```python
from build123d import *

# Parameters (mm, degrees)
SKETCH_1_W          = 15
SKETCH_1_H          = 15
SKETCH_1_W_2        = 12
SKETCH_1_H_2        = 12
EXTRUDE_1_DEPTH     = 267.5
SKETCH_2_R          = 2.15
CUT_EXTRUDE_1_DEPTH = 269.025185384
SKETCH_3_R          = 2.15
CUT_EXTRUDE_2_DEPTH = 269.025185384


with BuildPart() as part:
    # ｽｹｯﾁ1 → 押し出し-薄板1 (new body)
    with BuildSketch(Plane(origin=(0, 0, 0), x_dir=(1, 0, 0), z_dir=(0, 1, 0))):
        Rectangle(SKETCH_1_W, SKETCH_1_H)
        Rectangle(SKETCH_1_W_2, SKETCH_1_H_2, mode=Mode.SUBTRACT)
    extrude(amount=EXTRUDE_1_DEPTH)

    # ｽｹｯﾁ2 → ｶｯﾄ - 押し出し1 (cut, through all)
    with BuildSketch(Plane.ZY.offset(-7.5)):
        with Locations(Location((0, 5, 0), (0, 0, 180))):
            Circle(SKETCH_2_R)
        with Locations(Location((0, 262.5, 0), (0, 0, 180))):
            Circle(SKETCH_2_R)
        with Locations(Location((0, 250, 0), (0, 0, 180))):
            Circle(SKETCH_2_R)
    extrude(amount=CUT_EXTRUDE_1_DEPTH, mode=Mode.SUBTRACT)

    # ｽｹｯﾁ3 → ｶｯﾄ - 押し出し2 (cut, through all)
    with BuildSketch(Plane.XY.offset(7.5)):
        with Locations((0, 207.5)):
            Circle(SKETCH_3_R)
        with Locations((0, 232.5)):
            Circle(SKETCH_3_R)
        with Locations((0, 65)):
            Circle(SKETCH_3_R)
        with Locations((0, 40)):
            Circle(SKETCH_3_R)
    extrude(amount=-CUT_EXTRUDE_2_DEPTH, mode=Mode.SUBTRACT)


solid = part.part
```
The model under review builds one solid part; all positions refer to its coordinate system, in mm. A direction names the side the tool comes from. Give positions to 0.01 mm unless a question says otherwise; leave off trailing zeros. Write each loop counter-clockwise with the first axis right and the second up, starting at its lowest first coordinate (ties: lowest second). Pieces come first, ordered by that corner, then holes. Notation, with made-up numbers: (-8.75, -14.75) -> (50.25, -14.75) arc R29 cw to (50.25, 24.25) -> close; hole circle Ø10 at (73, -15.5). An arc over 180 degrees is marked (long way). Put each result on its own line as item: value.
(1) The part is to be moulded in two halves that separate along Z. For faces 1 (the flat face through (0, 132, 7.5)), 2 (the flat face through (-6, 132, 0)), 3 (the cylindrical face through (-0.28, 209.63, 6.76)), say which applies: pulls with the +Z half, pulls with the -Z half, needs draft (parallel to the pull), parting line crosses it, or undercut.
Results are:
face 1: pulls with the +Z half
face 2: undercut
face 3: needs draft
(2) We need section C-C, the plane x = 0. State how many separate pieces and enclosed holes the cut face has, and give its area (3 significant figures).
Results are:
separate pieces: 10
enclosed holes: 0
area: 751 mm²
(3) We need section B-B, the plane y = 30. Give the boundary of the cut face in (x, z), and give its area (3 significant figures).
Results are:
outline: (-7.5, -7.5) -> (7.5, -7.5) -> (7.5, 7.5) -> (-7.5, 7.5) -> close; hole (-6, -6) -> (6, -6) -> (6, 6) -> (-6, 6) -> close
area: 81.0 mm²
(4) To check wall thickness, follow probe 1 along Y at (x, z) = (0, 6.5); probe 2 along Z at (x, y) = (0.25, 191.5). State the ranges of each line that lie inside material, in increasing order. Write a range as from..to.
Results are:
probe 1: 0..37.85, 42.15..62.85, 67.15..205.35, 209.65..230.35, 234.65..267.5
probe 2: -7.5..-6, 6..7.5
(5) We need section A-A, the plane y = 207.5. Give the boundary of the cut face in (x, z), and give its area (3 significant figures).
Results are:
outline: (-7.5, -7.5) -> (-2.15, -7.5) -> (-2.15, -6) -> (-6, -6) -> (-6, 6) -> (-2.15, 6) -> (-2.15, 7.5) -> (-7.5, 7.5) -> close; (2.15, -7.5) -> (7.5, -7.5) -> (7.5, 7.5) -> (2.15, 7.5) -> (2.15, 6) -> (6, 6) -> (6, -6) -> (2.15, -6) -> close
area: 68.1 mm²
(6) Tool access review of faces 4 (the cylindrical face through (-0.28, 42.13, -6.74)), 5 (the flat face through (6, 132, 0)): name each direction out of +Z, -Z, +X, -X, +Y, -Y from which nothing blocks a thin tool from reaching the whole face with its end or side.
Results are:
face 4: +Z, -Z
face 5: +Y, -Y
